Autodesk Inventor part; units mm, degrees
ref_plane "YZ Plane" through (0, 0, 0) normal (1, 0, 0) x (0, 1, 0)
ref_plane "XZ Plane" through (0, 0, 0) normal (0, 1, 0) x (-1, 0, 0)
ref_plane "XY Plane" through (0, 0, 0) normal (0, 0, 1) x (1, 0, 0)
sketch "Sketch1" plane through (0, 0, 0) normal (0, 1, 0) x (-1, 0, 0)
  circle A0 centre (0, 0) radius 2.5
  dimension "d0" = 5
extrude "Extrusion1" add sketch "Sketch1" along normal blind 15
sketch "Sketch2" plane through (0, 15, 0) normal (0, 1, 0) x (1, 0, 0)
  circle A0 centre (0, 0) radius 2.5
  circle A1 centre (0, 0) radius 4.25
  dimension "d3" = 8.5
extrude "Extrusion2" add sketch "Sketch2" along normal blind 5 contours A0 | A1
sketch "Sketch3" plane through (0, 20, 0) normal (0, 1, 0) x (1, 0, 0)
  circle A0 centre (0, 0) radius 4.25
  line L0 (0, 2.3094) -> (2, 1.1547)
  line L1 (2, 1.1547) -> (2, -1.1547)
  line L2 (2, -1.1547) -> (0, -2.3094)
  line L3 (0, -2.3094) -> (-2, -1.1547)
  line L4 (-2, -1.1547) -> (-2, 1.1547)
  line L5 (-2, 1.1547) -> (0, 2.3094)
  dimension "d6" = 2
extrude "Extrusion3" cut sketch "Sketch3" against normal blind 3.2 contours L0 L1 L2 L3 L4 L5
thread "Thread1"
chamfer "Chamfer1" distance 0.25 angle 45 1 edges at (2.5, 0, 0)
properties part number "SHCS5x15" material "Stainless Steel"
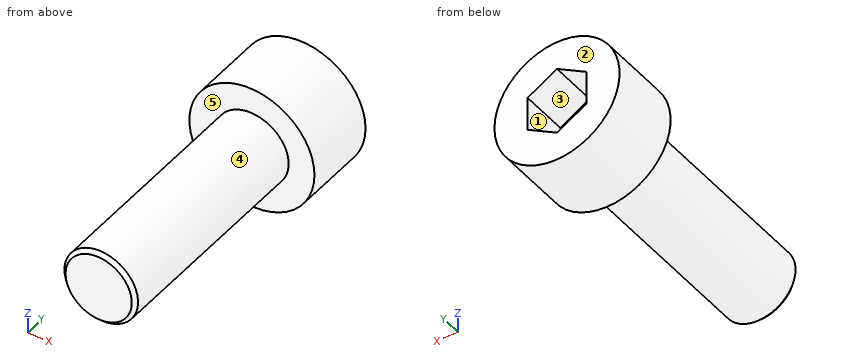
Can you work these out from the model? Positions are in its coordinate system, mm. Face numbers are marked on the shaded views. A direction names the side the tool comes from. Round coordinates to 2 decimals unless told otherwise and drop trailing zeros. Loops run counter-clockwise (first coordinate to the right, second up) from the corner with the lowest first, then second, coordinate; pieces in that order, holes last.
Item 1: Suppose I cut it at B-B, the plane z = 0. Write out the boundary of the cut face in (x, y), then the cut area to 3 significant figures.
Item 2: Suppose I cut it at D-D, the plane x = 2.75. Write out the boundary of the cut face in (y, z), then the cut area to 3 significant figures.
Item 3: Please list where these lines run through material, in increasing order: L1, parallel to X at y = 17.75, z = 3.75; L2, parallel to Y at x = -1, z = 0.5; L3, parallel to X at y = 17.25, z = 1.5.
Item 4: Which directions (+Z, -Z, +X, -X, +Y, -Y) give clear straight access to the entire face, cutting with the end or side of a thin tool? Please do the marked faces 1 and 2.
Item 5: If we mould it in two halves opening along X, with no side actions, what happens to the marked faces 3, 4 and 5? For each: +X half, -X half, draft (parallel to the pull), parting line (faces both ways), or undercut.
Item 6: Suppose I cut it at C-C, the plane y = 12.25. Write out the boundary of the cut face in (x, z).
Item 7: Will these pins go through, and if not, where does the flat tip stop? pin 1 Ø3 at (y, z) = (5.5, 2) entering from +X; pin 2 Ø1.5 at (x, z) = (1.5, -2.5) entering from -Y; pin 3 Ø2 at (x, z) = (-0.5, -3.5) entering from -Y; pin 4 Ø2 at (x, y) = (-2, 2) entering from -Z.
Item 8: Suppose I cut it at A-A, the plane y = 18.5. Write out the boundary of the cut face in (x, z).
Reported:
1. outline: (-4.25, 15) - (-2.5, 15) - (-2.5, 0.25) - (-2.25, 0) - (2.25, 0) - (2.5, 0.25) - (2.5, 15) - (4.25, 15) - (4.25, 20) - (2, 20) - (2, 16.8) - (-2, 16.8) - (-2, 20) - (-4.25, 20) - close
1. area: 105 mm2
2. outline: (15, -3.24) - (20, -3.24) - (20, 3.24) - (15, 3.24) - close
2. area: 32.4 mm2
3. L1: x = -2 to 2
3. L2: y = 0 to 16.8
3. L3: x = -3.98 to -1.4, 1.4 to 3.98
4. face 1: +Y
4. face 2: +Z, -Z, +X, -X, +Y
5. face 3: undercut
5. face 4: parting line
5. face 5: draft
6. outline: circle Ø5 at (0, 0)
7. pin 1: stops at x = 2.45
7. pin 2: stops at y = 0
7. pin 3: stops at y = 15
7. pin 4: stops at z = -2.29
8. outline: circle Ø8.5 at (0, 0); hole (-2, -1.15) - (0, -2.31) - (2, -1.15) - (2, 1.15) - (0, 2.31) - (-2, 1.15) - close
